Here's how the part is built. I have some questions about the finished solid (model axes, mm). Face numbers are marked on the shaded views. Give positions to 0.01 mm unless a question says otherwise; leave off trailing zeros. Order: outer loops, then holes, each group sorted by start corner. A loop starts at its lowest first (then second) coordinate and runs counter-clockwise, first axis right, second up.
from build123d import *

# Parameters (mm, degrees)
F0_R     = 32.5
F1_DEPTH = 5
F2_D     = 15
F3_D     = 5
F4_D     = 2.5
F4_DEPTH = 10
F4_TIP   = 0.7510757738


with BuildPart() as f1:
    # F0 (on Top) → F1 (new body)
    with BuildSketch(Plane.XY):
        Circle(F0_R)
    extrude(amount=F1_DEPTH)

    # F2 (through all)
    with Locations(Plane(origin=(0, 0, 0), x_dir=(1, 0, 0), z_dir=(0, 0, -1))):
        with Locations((19.0525588833, -11), (0, -22), (-19.0525588833, -11), (-19.0525588833, 11), (0, 22), (19.0525588833, 11)):
            Hole(F2_D / 2)

    # F3 (through all)
    with Locations(Plane(origin=(0, 0, 0), x_dir=(1, 0, 0), z_dir=(0, 0, -1))):
        with Locations((-8.6602540378, 5), (0, -10), (8.6602540378, 5)):
            Hole(F3_D / 2)

    # F4
    with Locations(Plane(origin=(0, 0, 0), x_dir=(1, 0, 0), z_dir=(0, 0, -1))):
        with Locations((0, 0)):
            Hole(F4_D / 2, depth=F4_DEPTH)
            with Locations((0, 0, -(F4_DEPTH + F4_TIP / 2))):  # 118° drill point
                Cone(0, F4_D / 2, F4_TIP, mode=Mode.SUBTRACT)


solid = f1.part
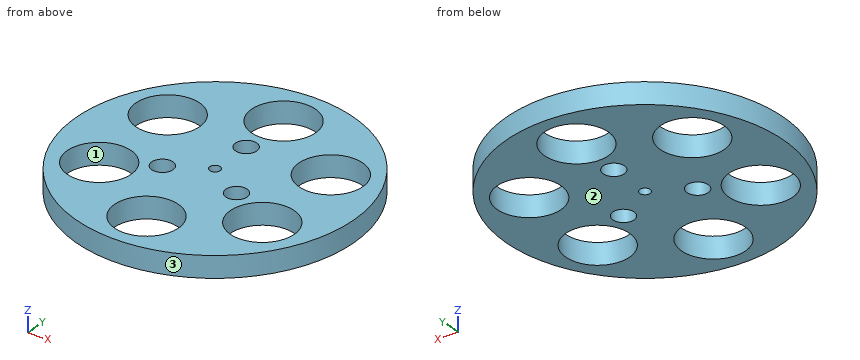
Q1. I'm going to push flat-ended pins straight in: P1, Ø1, axis at y = 12, z = 3.5, coming from the -X side; P2, Ø12, axis at x = -19.05, y = -11, coming from the +Z side; P3, Ø12, axis at x = -14, y = 15.5, coming from the +Z side; P4, Ø1.5, axis at y = -7, z = 3.5, coming from the +X side. Where does each tip first touch, or does it pass through?
Filled sheet:
P1: stops at x = -30.4
P2: passes through
P3: stops at z = 5
P4: stops at x = 31.89
Q2. Thinking about a two-plate mould opening in X: for the marked faces 1, 2 and 3, which applies, released by +X, released by -X, zero draft, split by the parting line, or undercut?
Filled sheet:
face 1: undercut
face 2: zero draft
face 3: split by the parting line
Q3. If we section it at B-B on x = 0: List the corners of the cut face in (y, z) for me, plus the area to 4 significant figures.
Filled sheet:
outline: (-32.5, 0) - (-29.5, 0) - (-29.5, 5) - (-32.5, 5) - close; (-14.5, 0) - (-1.25, 0) - (-1.25, 5) - (-14.5, 5) - close; (1.25, 0) - (7.5, 0) - (7.5, 5) - (1.25, 5) - close; (12.5, 0) - (14.5, 0) - (14.5, 5) - (12.5, 5) - close; (29.5, 0) - (32.5, 0) - (32.5, 5) - (29.5, 5) - close
area: 137.5 mm2
Q4. If we section it at D-D on y = -9: List the corners of the cut face in (x, z) for me, plus the area to 3 significant figures.
Filled sheet:
outline: (-31.23, 0) - (-26.28, 0) - (-26.28, 5) - (-31.23, 5) - close; (-11.82, 0) - (11.82, 0) - (11.82, 5) - (-11.82, 5) - close; (26.28, 0) - (31.23, 0) - (31.23, 5) - (26.28, 5) - close
area: 168 mm2
Q5. If we section it at C-C on z = 3.7: Give the number of separate pieces and of enclosed holes in the cut face, plus the area to 3 significant figures.
Filled sheet:
separate pieces: 1
enclosed holes: 10
area: 2,190 mm2
Q6. I need wall thicknesses on L1, parallel to X at y = -14, z = 2.5; L2, parallel to X at y = 10, z = 4; L3, parallel to Y at x = -2, z = 0.65. Which ranges of each line are inside material? Lowest first, please.
Filled sheet:
L1: x = -29.33 to -25.93, -12.18 to 12.18, 25.93 to 29.33
L2: x = -30.92 to -26.49, -11.62 to -2.5, 2.5 to 11.62, 26.49 to 30.92
L3: y = -32.44 to -29.23, -14.77 to 8.5, 11.5 to 14.77, 29.23 to 32.44
Q7. If we section it at A-A on y = 0: List the corners of the cut face in (x, z) for me.
Filled sheet:
outline: (-32.5, 0) - (-1.25, 0) - (-1.25, 5) - (-32.5, 5) - close; (1.25, 0) - (32.5, 0) - (32.5, 5) - (1.25, 5) - close
